Autodesk Inventor part; units mm, degrees
ref_plane "YZ Plane" through (0, 0, 0) normal (1, 0, 0) x (0, 1, 0)
ref_plane "XZ Plane" through (0, 0, 0) normal (0, 1, 0) x (-1, 0, 0)
ref_plane "XY Plane" through (0, 0, 0) normal (0, 0, 1) x (1, 0, 0)
sketch "Sketch1" plane through (0, 0, 0) normal (0, 0, 1) x (1, 0, 0)
  line L0 (0, 0) -> (-65, 0)
  line L1 (-65, 0) -> (-65, 65)
  line L2 (-65, 65) -> (0, 65)
  line L3 (0, 65) -> (0, 0)
  dimension "d4" = 65
  dimension "d5" = 65
extrude "Extrusion1" add sketch "Sketch1" along normal blind 10
sketch "Sketch2" plane through (0, 0, 10) normal (0, 0, 1) x (1, 0, 0)
  line L0 (-5, 5) -> (-60, 5)
  line L1 (-60, 5) -> (-60, 60)
  line L2 (-60, 60) -> (-5, 60)
  line L3 (-5, 60) -> (-5, 5)
  point P0 (0, 0)
  dimension "d8" = 55
  dimension "d9" = 55
extrude "Extrusion2" cut sketch "Sketch2" against normal blind 2
sketch "Sketch3" plane through (0, 0, 0) normal (0, 0, -1) x (-1, 0, 0)
  line L0 (30, 35) -> (35, 35)
  line L1 (35, 35) -> (35, 30)
  line L2 (35, 30) -> (30, 30)
  line L3 (30, 30) -> (30, 35)
  point P0 (0, 0)
  point P1 (32.5, 32.5)
  dimension "d20" = 5
  dimension "d21" = 5
extrude "Extrusion4" cut sketch "Sketch3" against normal blind 5
properties part number "Clip_MarkerHolderV1"
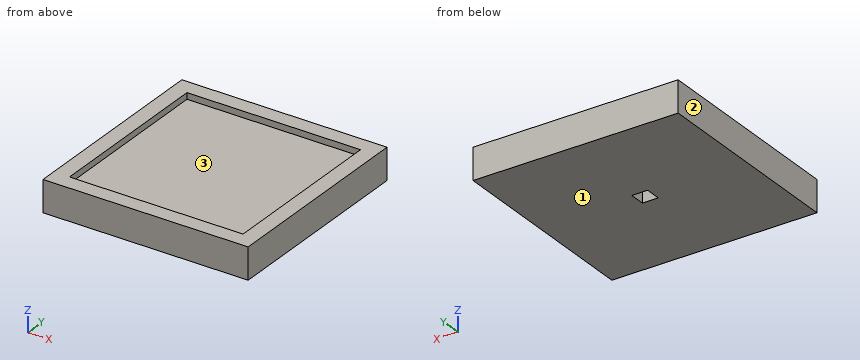
Here's how the part is built. I have some questions about the finished solid (model axes, mm). Face numbers are marked on the shaded views. Coordinates: 2 decimals unless noted, no trailing zeros. Order: outer loops, then holes, each group sorted by start corner. A loop starts at its lowest first (then second) coordinate and runs counter-clockwise, first axis right, second up. Notation, with made-up numbers: (72.25, 22) -> (96.25, 22) arc R11 ccw to (96.25, 35) -> close; hole circle Ø8 at (19, 38). An arc over 180 degrees is marked (long way). Answer in a Markdown table with one row per item.
(1) Please list where these lines run through material, in increasing order: probe 1 along X at (y, z) = (45, 8.25); probe 2 along Z at (x, y) = (-14, 51); probe 3 along X at (y, z) = (33.5, 1).
Answer key:
| item | result |
|---|---|
| probe 1 | -65 to -60, -5 to 0 |
| probe 2 | 0 to 8 |
| probe 3 | -65 to -35, -30 to 0 |
(2) Will these pins go through, and if not, where does the flat tip stop? pin 1 Ø1.5 at (x, y) = (-14.5, 17) entering from +Z; pin 2 Ø1.5 at (x, y) = (-32, 32) entering from -Z.
Answer key:
| item | result |
|---|---|
| pin 1 | z = 8 |
| pin 2 | z = 5 |
(3) I want a section at C-C on x = -32. List the corners of the cut face in (y, z) for me, then the cut area to 3 significant figures.
Answer key:
| item | result |
|---|---|
| outline | (0, 0) -> (30, 0) -> (30, 5) -> (35, 5) -> (35, 0) -> (65, 0) -> (65, 10) -> (60, 10) -> (60, 8) -> (5, 8) -> (5, 10) -> (0, 10) -> close |
| area | 515 mm^2 |
(4) Thinking about a two-plate mould opening in X: for the marked faces 1, 2 and 3, which applies, +X half, -X half, draft (parallel to the pull), parting line (faces both ways), or undercut?
Answer key:
| item | result |
|---|---|
| face 1 | draft |
| face 2 | -X half |
| face 3 | undercut |
(5) I want a section at B-B on y = 40. List the corners of the cut face in (x, z) for me.
Answer key:
| item | result |
|---|---|
| outline | (-65, 0) -> (0, 0) -> (0, 10) -> (-5, 10) -> (-5, 8) -> (-60, 8) -> (-60, 10) -> (-65, 10) -> close |
(6) I want a section at A-A on x = -52. List the corners of the cut face in (y, z) for me.
Answer key:
| item | result |
|---|---|
| outline | (0, 0) -> (65, 0) -> (65, 10) -> (60, 10) -> (60, 8) -> (5, 8) -> (5, 10) -> (0, 10) -> close |
